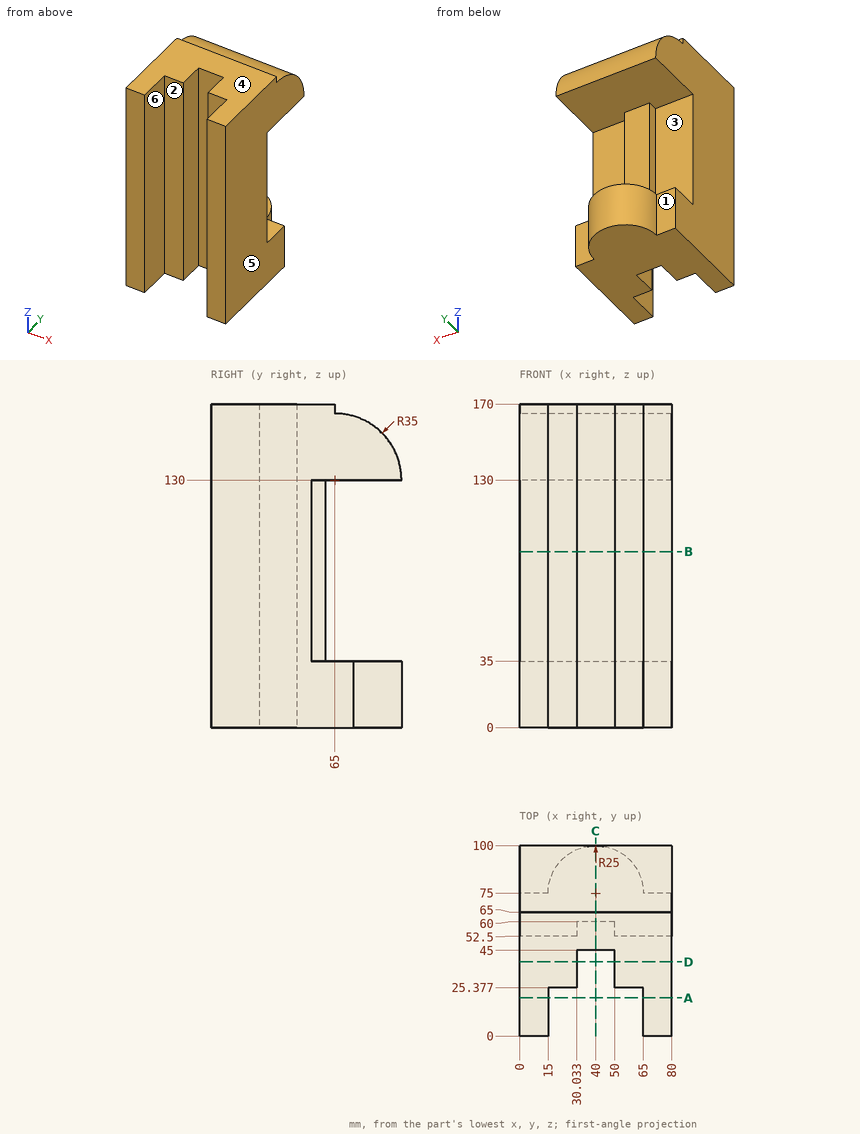
Job drawing, mm, ordinate dimensions from the low corner. One solid piece. A direction names the side the tool comes from. Round coordinates to 2 decimals unless told otherwise and drop trailing zeros. Loops run counter-clockwise (first coordinate to the right, second up) from the corner with the lowest first, then second, coordinate; pieces in that order, holes last. Notation, with made-up numbers: (28, -31.75) -> (40, -31.75) arc R11 cw to (40, -10.75) -> close; hole circle Ø4 at (43, 77). An arc over 180 degrees is marked (long way). One line per item, written item: value. Start each with the question number.
Q1. Cut at C-C on x = 40. List the corners of the cut face in (y, z).
Q2. Two-plate mould, pull along X, no slides. Class the marked faces 4, 5 and 6: released by +X, released by -X, zero draft, split by the parting line, or undercut.
Q3. 3-axis set-ups, long thin cutter, end or side, ignore diameter. For the marked faces 1, 2 and 3: which of +Z, -Z, +X, -X, +Y, -Y reach the whole face in a straight line?
Q4. Cut at A-A on y = 20. List the corners of the cut face in (x, z), plus the area to 3 significant figures.
Q5. Cut at D-D on y = 39. List the corners of the cut face in (x, z).
Q6. Probe line 1 along Z through (x, y) = (60, 64); line 2 along X through (y, z) = (30, 7); line 3 along X through (y, z) = (4.5, 138). List the from-to ranges inside material, lowest first.
Q7. Drop flat-ended pins along their axis: pin 1 Ø12 at (x, y) = (57.5, 16) entering from -Z; pin 2 Ø8 at (y, z) = (57, 93) entering from +X; pin 3 Ø7.5 at (x, z) = (54, 118.5) entering from -Y; pin 4 Ø22 at (x, z) = (38, 59) entering from +Y. Give the stop position or say it passes through.
Q8. Cut at B-B on z = 92.5. List the corners of the cut face in (x, y), plus the area to 3 significant figures.
Computed:
1. outline: (45, 0) -> (100, 0) -> (100, 35) -> (60, 35) -> (60, 130) -> (100, 130) arc R35 ccw to (65, 165) -> (65, 170) -> (45, 170) -> close
2. face 4: zero draft
2. face 5: released by +X
2. face 6: undercut
3. face 1: -Z, -X, +Y
3. face 2: +Z, -Z, -Y
3. face 3: -X, +Y
4. outline: (0, 0) -> (15, 0) -> (15, 170) -> (0, 170) -> close; (65, 0) -> (80, 0) -> (80, 170) -> (65, 170) -> close
4. area: 5,100 mm²
5. outline: (0, 0) -> (30.03, 0) -> (30.03, 170) -> (0, 170) -> close; (50, 0) -> (80, 0) -> (80, 170) -> (50, 170) -> close
6. line 1: 0 to 35, 130 to 170
6. line 2: 0 to 30.03, 50 to 80
6. line 3: 0 to 15, 65 to 80
7. pin 1: through
7. pin 2: x = 50
7. pin 3: y = 25.38
7. pin 4: y = 60
8. outline: (0, 0) -> (15, 0) -> (15, 25.38) -> (30.03, 25.38) -> (30.03, 45) -> (50, 45) -> (50, 25.38) -> (65, 25.38) -> (65, 0) -> (80, 0) -> (80, 52.5) -> (50, 52.5) -> (50, 60) -> (30.03, 60) -> (30.03, 52.5) -> (0, 52.5) -> close
8. area: 2,690 mm²
